Source: CAD feature listing. Evaluate the final solid. Frame: model axes, mm. A direction names the side the tool comes from. Give positions to 0.01 mm unless a question says otherwise; leave off trailing zeros. Loops run counter-clockwise (first coordinate to the right, second up) from the corner with the lowest first, then second, coordinate; pieces in that order, holes last. Notation, with made-up numbers: (-32.5, 13.5) -> (9.5, 13.5) arc R24 ccw to (9.5, 46.5) -> close; hole circle Ø10 at (-4, -35). An arc over 180 degrees is marked (long way). Answer as a JSON object with one key per item and string values. Group by question number.
from build123d import *

# Parameters (mm, degrees)
SKETCH_1_R          = 12
SKETCH_1_W          = 30
SKETCH_1_H          = 145
EXTRUDE_1_DEPTH     = 12
SKETCH_2_W          = 30
SKETCH_2_H          = 50
EXTRUDE_2_DEPTH     = 10
SKETCH_3_R          = 10.9
CUT_EXTRUDE_1_DEPTH = 3
SKETCH_4_R          = 1.675
CUT_EXTRUDE_2_DEPTH = 18
CHAMFER_1_SIZE      = 15
SKETCH_5_R          = 10.75
CUT_EXTRUDE_3_DEPTH = 1
SKETCH_8_R          = 1.6
CUT_EXTRUDE_4_DEPTH = 14
SKETCH_9_R          = 1.325
CUT_EXTRUDE_5_DEPTH = 120
SKETCH_10_R         = 1.275
CUT_EXTRUDE_6_DEPTH = 120
SKETCH_11_R         = 1.65
CUT_EXTRUDE_7_DEPTH = 130
SKETCH_12_R         = 1.65
CUT_EXTRUDE_8_DEPTH = 120


with BuildPart() as part:
    # 草图1 → 凸台-拉伸1 (new body)
    with BuildSketch(Plane.XY.offset(38)):
        Circle(SKETCH_1_R)
        with Locations((0, 72.5)):
            Rectangle(SKETCH_1_W, SKETCH_1_H)
        with BuildLine():
            ThreePointArc((12, 0), (0, 12), (-12, 0))
            Line((-12, 0), (12, 0))
        make_face()
        with BuildLine():
            Line((12, 0), (-12, 0))
            ThreePointArc((-12, 0), (0, -12), (12, 0))
        make_face()
    extrude_1 = extrude(amount=EXTRUDE_1_DEPTH)

    # 草图2 → 凸台-拉伸2 (add)
    with BuildSketch(Plane(origin=(0, 145, 0), x_dir=(1, 0, 0), z_dir=(0, 1, 0))):
        with Locations((0, -25)):
            Rectangle(SKETCH_2_W, SKETCH_2_H)
    extrude_2 = extrude(amount=EXTRUDE_2_DEPTH)

    # 草图3 → 切除-拉伸1 (cut)
    with BuildSketch(Plane(origin=(0, 0, 38), x_dir=(-1, 0, 0), z_dir=(0, 0, -1))):
        Circle(SKETCH_3_R)
    cut_extrude_1 = extrude(amount=-CUT_EXTRUDE_1_DEPTH, mode=Mode.SUBTRACT)

    # 草图4 → 切除-拉伸2 (cut, symmetric)
    with BuildSketch(Plane(origin=(0, 0, 41), x_dir=(-1, 0, 0), z_dir=(0, 0, -1))):
        Circle(SKETCH_4_R)
    cut_extrude_2 = extrude(amount=CUT_EXTRUDE_2_DEPTH, both=True, mode=Mode.SUBTRACT)

    # 镜向1: 凸台-拉伸2 across plane
    add(extrude_2.mirror(Plane.XY))

    # 镜向2: 凸台-拉伸1, 切除-拉伸1, 切除-拉伸2 across plane
    add(extrude_1.mirror(Plane.XY))
    add(cut_extrude_1.mirror(Plane.XY), mode=Mode.SUBTRACT)
    add(cut_extrude_2.mirror(Plane.XY), mode=Mode.SUBTRACT)

    # 倒角1
    chamfer_1_edges = [part.edges().sort_by_distance(p)[0] for p in [
        (0, 155, 50),
        (0, 155, -50),
        (0, 145, -38),
        (0, 145, 38),
    ]]
    chamfer(chamfer_1_edges, length=CHAMFER_1_SIZE)

    # 草图5 → 切除-拉伸3 (cut)
    with BuildSketch(Plane(origin=(0, 155, 0), x_dir=(1, 0, 0), z_dir=(0, 1, 0))):
        with Locations(Location((0, 0, 0), (0, 0, 180))):
            Circle(SKETCH_5_R)
    extrude(amount=-CUT_EXTRUDE_3_DEPTH, mode=Mode.SUBTRACT)

    # 草图8 → 切除-拉伸4 (cut)
    with BuildSketch(Plane(origin=(0, 154, 0), x_dir=(1, 0, 0), z_dir=(0, 1, 0))):
        with Locations(Location((0, 0, 0), (0, 0, 180))):
            Circle(SKETCH_8_R)
    extrude(amount=-CUT_EXTRUDE_4_DEPTH, mode=Mode.SUBTRACT)

    # 草图9 → 切除-拉伸5 (cut)
    with BuildSketch(Plane.XY.offset(50)):
        with Locations((-7, 0)):
            Circle(SKETCH_9_R)
        with Locations((0, 7)):
            Circle(SKETCH_9_R)
        with Locations((7, 0)):
            Circle(SKETCH_9_R)
        with Locations((0, -7)):
            Circle(SKETCH_9_R)
    extrude(amount=-CUT_EXTRUDE_5_DEPTH, mode=Mode.SUBTRACT)

    # 草图10 → 切除-拉伸6 (cut)
    with BuildSketch(Plane(origin=(0, 155, 0), x_dir=(1, 0, 0), z_dir=(0, 1, 0))):
        with Locations(Location((-7, 0, 0), (0, 0, 180))):
            Circle(SKETCH_10_R)
        with Locations(Location((0, 7, 0), (0, 0, 180))):
            Circle(SKETCH_10_R)
        with Locations(Location((7, 0, 0), (0, 0, 180))):
            Circle(SKETCH_10_R)
        with Locations(Location((0, -7, 0), (0, 0, 180))):
            Circle(SKETCH_10_R)
    extrude(amount=-CUT_EXTRUDE_6_DEPTH, mode=Mode.SUBTRACT)

    # 草图11 → 切除-拉伸7 (cut)
    with BuildSketch(Plane.XY.offset(50)):
        with Locations(Location((-5, 30, 0), (0, 0, 180))):
            Circle(SKETCH_11_R)
        with Locations(Location((5, 30, 0), (0, 0, 180))):
            Circle(SKETCH_11_R)
        with Locations(Location((-5, 90, 0), (0, 0, 180))):
            Circle(SKETCH_11_R)
        with Locations(Location((5, 90, 0), (0, 0, 180))):
            Circle(SKETCH_11_R)
    extrude(amount=-CUT_EXTRUDE_7_DEPTH, mode=Mode.SUBTRACT)

    # 草图12 → 切除-拉伸8 (cut)
    with BuildSketch(Plane.XY.offset(50)):
        with Locations(Location((-5, 65, 0), (0, 0, 180))):
            Circle(SKETCH_12_R)
        with Locations(Location((5, 65, 0), (0, 0, 180))):
            Circle(SKETCH_12_R)
    extrude(amount=-CUT_EXTRUDE_8_DEPTH, mode=Mode.SUBTRACT)


solid = part.part
(1) Section query A-A on y = 112.5. Return the cut outline in (x, z).
(2) Mould query, pull axis Y, two halves, no side actions, for faces 5 (the face through (0, 148, -42)), 6 (the face through (13, 0, 44)), 7 (the face through (-4.785, 28.364, 44.084)), 8 (the face through (15, 89, 41)). Classes: pulls with the +Y half, pulls with the -Y half, needs draft (parallel to the pull), parting line crosses it, or undercut.
(3) Section query B-B on y = 65. Return the cut outline in (x, z).
(4) Access query for faces 1 (the face through (5.4, 91.6, 44.1)), 2 (the face through (0, 137, 31)), 3 (the face through (0, -2, 41)), 4 (the face through (-14, 0, -44)). Directions: +Z, -Z, +X, -X, +Y, -Y. A direction counts if a zero-diameter tool reaches every point of the face in a straight line with its end or side. Return the directions, or none.
(5) Section query C-C on z = -26.5. Return the cut outline in (x, y).
(6) First-contact query: pin 1 (1.5 mm diameter, centred on x = 6, z = 2.5, fed in from -Y). Flat tip, straight axial feed; report the tip coordinate or a pass-through.
(7) Section query D-D on z = 15. Return the cut outline in (x, y).
(8) Material intervals for line 1 (X direction, y = 30, z = -46); line 2 (Z direction, x = 4, y = 20); line 3 (Y direction, x = -5, z = 45), sorted ascending. Write a range as from..to.
Result:
{
 "1": {"outline": "(-15, -50) -> (15, -50) -> (15, -38) -> (-15, -38) -> close; (-15, 38) -> (15, 38) -> (15, 50) -> (-15, 50) -> close"},
 "2": {"face 5": "pulls with the +Y half", "face 6": "pulls with the -Y half", "face 7": "undercut", "face 8": "needs draft"},
 "3": {"outline": "(-15, -50) -> (-6.65, -50) -> (-6.65, -38) -> (-15, -38) -> close; (-15, 38) -> (-6.65, 38) -> (-6.65, 50) -> (-15, 50) -> close; (-3.35, -50) -> (3.35, -50) -> (3.35, -38) -> (-3.35, -38) -> close; (-3.35, 38) -> (3.35, 38) -> (3.35, 50) -> (-3.35, 50) -> close; (6.65, -50) -> (15, -50) -> (15, -38) -> (6.65, -38) -> close; (6.65, 38) -> (15, 38) -> (15, 50) -> (6.65, 50) -> close"},
 "4": {"face 1": "+Z, -Z", "face 2": "+X, -X, -Y", "face 3": "none", "face 4": "+Z, -Z, -X, -Y"},
 "5": {"outline": "(-15, 141.5) -> (15, 141.5) -> (15, 155) -> (-15, 155) -> close"},
 "6": {"pin 1": "y = 145"},
 "7": {"outline": "(-15, 145) -> (15, 145) -> (15, 155) -> (-15, 155) -> close"},
 "8": {"line 1": "-15..-6.65, -3.35..3.35, 6.65..15", "line 2": "-50..-38, 38..50", "line 3": "-10.91..28.35, 31.65..63.35, 66.65..88.35, 91.65..145"}
}
